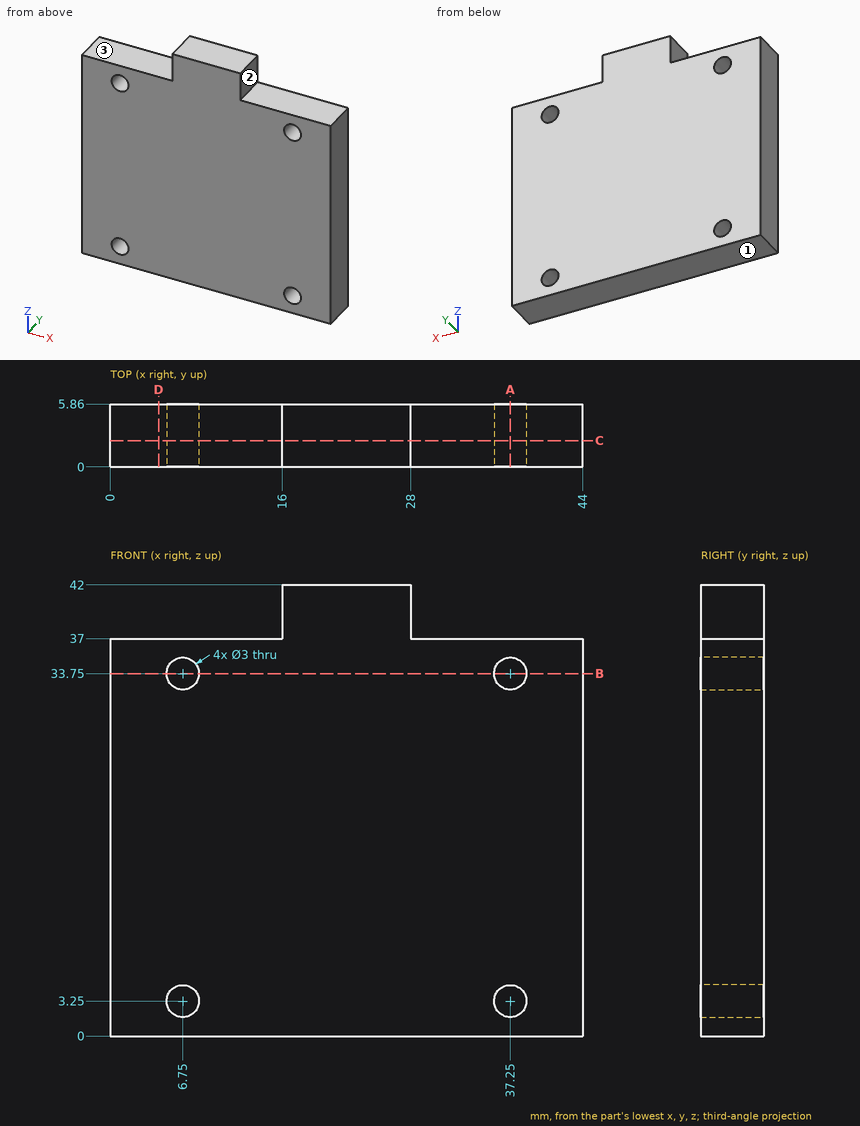
Could you check a few things on this drawing? It's one solid part, dimensions in mm from its lowest x, y, z. A direction names the side the tool comes from. Round coordinates to 2 decimals unless told otherwise and drop trailing zeros. Order: outer loops, then holes, each group sorted by start corner. A loop starts at its lowest first (then second) coordinate and runs counter-clockwise, first axis right, second up.
(1) Imagine slicing it at A-A (x = 37.25). Write out the boundary of the cut face in (y, z).
Response values:
outline: (0, 0) - (5.86, 0) - (5.86, 1.75) - (0, 1.75) - close; (0, 4.75) - (5.86, 4.75) - (5.86, 32.25) - (0, 32.25) - close; (0, 35.25) - (5.86, 35.25) - (5.86, 37) - (0, 37) - close
(2) Imagine slicing it at D-D (x = 4.5). Write out the boundary of the cut face in (y, z).
Response values:
outline: (0, 0) - (5.86, 0) - (5.86, 37) - (0, 37) - close
(3) I'm going to push flat-ended pins straight in: pin 1 (1.5 mm diameter, centred on y = 3.5, z = 38.5, fed in from +X); pin 2 (12 mm diameter, centred on x = 7.5, z = 12.5, fed in from -Y). Where does each tip first touch, or does it pass through?
Response values:
pin 1: stops at x = 28
pin 2: stops at y = 0
(4) Which directions (+Z, -Z, +X, -X, +Y, -Y) give clear straight access to the entire face, cutting with the end or side of a thin tool? Please do the marked faces 1, 2 and 3.
Response values:
face 1: -Z, +X, -X, +Y, -Y
face 2: +Z, +X, +Y, -Y
face 3: +Z, -X, +Y, -Y
(5) Imagine slicing it at B-B (z = 33.75). Write out the boundary of the cut face in (x, y), plus the area to 3 significant figures.
Response values:
outline: (0, 0) - (5.25, 0) - (5.25, 5.86) - (0, 5.86) - close; (8.25, 0) - (35.75, 0) - (35.75, 5.86) - (8.25, 5.86) - close; (38.75, 0) - (44, 0) - (44, 5.86) - (38.75, 5.86) - close
area: 223 mm2
(6) Imagine slicing it at C-C (y = 2.45). Write out the boundary of the cut face in (x, z), plus the area to 3 significant figures.
Response values:
outline: (0, 0) - (44, 0) - (44, 37) - (28, 37) - (28, 42) - (16, 42) - (16, 37) - (0, 37) - close; hole circle Ø3 at (6.75, 3.25); hole circle Ø3 at (6.75, 33.75); hole circle Ø3 at (37.25, 3.25); hole circle Ø3 at (37.25, 33.75)
area: 1,660 mm2
(7) Please list where these lines run through material, in increasing order: line 1 along Z through (x, y) = (6.75, 1.25); line 2 along X through (y, z) = (4.45, 3.25); line 3 along Z through (x, y) = (36, 0.35).
Response values:
line 1: z = 0 to 1.75, 4.75 to 32.25, 35.25 to 37
line 2: x = 0 to 5.25, 8.25 to 35.75, 38.75 to 44
line 3: z = 0 to 2.42, 4.08 to 32.92, 34.58 to 37
